```python
from build123d import *

# Parameters (mm, degrees)
F1_DEPTH = 43


with BuildPart() as f1:
    # F0 (on Top) → F1 (new body)
    with BuildSketch(Plane.XY):
        with BuildLine():
            Line((-14, 11), (-14, -7))
            Line((-14, -7), (-7, -14))
            Line((-7, -14), (0, -14))
            Line((0, -14), (21.066626, -14))
            ThreePointArc((21.066626, -14), (24.331862, -15.213414), (26.012265, -18.264706))
            ThreePointArc((26.012265, -18.264706), (28.349095, -26.115672), (32.788067, -33))
            Line((32.788067, -33), (38, -33))
            Line((38, -33), (67, 0))
            Line((67, 0), (67, 19))
            Line((67, 19), (62, 24))
            Line((62, 24), (38, 24))
            ThreePointArc((38, 24), (29.574973, 16.276069), (18.243085, 14.783252))
            Line((18.243085, 14.783252), (0, 18))
            Line((0, 18), (-7, 18))
            Line((-7, 18), (-14, 11))
        make_face()
        with BuildLine():
            ThreePointArc((7, 0), (4.949747, -4.949747), (0, -7))
            ThreePointArc((0, -7), (-4.949747, 4.949747), (7, 0))
        make_face(mode=Mode.SUBTRACT)
    extrude(amount=F1_DEPTH)


solid = f1.part
```
Build history of the part. All positions in model axes, mm. A direction names the side the tool comes from. Coordinates: 2 decimals unless noted, no trailing zeros. Order: outer loops, then holes, each group sorted by start corner. A loop starts at its lowest first (then second) coordinate and runs counter-clockwise, first axis right, second up. Notation, with made-up numbers: (49.25, 79.5) -> (62.25, 79.5) arc R33 cw to (62.25, 108.5) -> close; hole circle Ø11 at (49, 6.25). An arc over 180 degrees is marked (long way). Answer in a Markdown table with one row per item. Add a question column.
Q1. Band-saw the part on D-D, the plane x = 52.5. List the corners of the cut face in (y, z), then the cut area to 3 significant figures.
Q2. Band-saw the part on A-A, the plane z = 3. List the corners of the cut face in (x, y).
Q3. Drop flat-ended pins along their axis: pin 1 (3 mm diameter, centred on y = -6.5, z = 11.5, fed in from +X); pin 2 (3 mm diameter, centred on y = -26.5, z = 8, fed in from +X); pin 3 (10 mm diameter, centred on x = 12.5, z = 5, fed in from +Y); pin 4 (18 mm diameter, centred on x = 0, y = 0, fed in from +Z). Give the stop position or say it passes through.
Q4. Band-saw the part on C-C, the plane x = 6. List the corners of the cut face in (y, z), then the cut area to 3 significant figures.
Q5. Wall check: line 1 along Y through (x, z) = (0, 12); line 2 along Y through (x, z) = (0.5, 34.5); line 3 along X through (y, z) = (1, 35.5). Give the ranges that are in metal, low to high. Write a range as [from, to].
Q6. Band-saw the part on B-B, the plane y = -6. List the corners of the cut face in (x, z), then the cut area to 3 significant figures.
Q7. Which spindle directions (+Z, -Z, +X, -X, +Y, -Y) get a long thin tool onto all of the face, cutting with end or side? Do faces 1 (the face through (-14, 2, 21)), 2 (the face through (-3, 18, 21)), 3 (the face through (52.3, -16.73, 21.2)), 4 (the face through (9.25, 16.37, 21.2)), 5 (the face through (7, -14, 21)). Say none if no direction does.
Q8. Mould opens along X. For faces 6 (the face through (26, 2, 43)), 7 (the face through (24.29, -15.18, 21.2)), 8 (the face through (29.722, 16.345, 21.199)) say: +X half, -X half, draft (parallel to the pull), parting line (faces both ways), or undercut.
Answers follow:
| question | item | result |
|---|---|---|
| 1 | outline | (-16.5, 0) -> (24, 0) -> (24, 43) -> (-16.5, 43) -> close |
| 1 | area | 1,740 mm^2 |
| 2 | outline | (-14, -7) -> (-7, -14) -> (21.07, -14) arc R5 cw to (26.01, -18.26) arc R29 ccw to (32.79, -33) -> (38, -33) -> (67, 0) -> (67, 19) -> (62, 24) -> (38, 24) arc R19 cw to (18.24, 14.78) -> (0, 18) -> (-7, 18) -> (-14, 11) -> close; hole (0, -7) arc R7 ccw to (7, 0) arc R7 ccw (long way) to start |
| 3 | pin 1 | x = 62.61 |
| 3 | pin 2 | x = 45.03 |
| 3 | pin 3 | y = 16.68 |
| 3 | pin 4 | z = 43 |
| 4 | outline | (-14, 0) -> (-3.61, 0) -> (-3.61, 43) -> (-14, 43) -> close; (3.61, 0) -> (16.94, 0) -> (16.94, 43) -> (3.61, 43) -> close |
| 4 | area | 1,020 mm^2 |
| 5 | line 1 | [-14, -7], [7, 18] |
| 5 | line 2 | [-14, -6.98], [6.98, 17.91] |
| 5 | line 3 | [-14, -6.93], [6.93, 67] |
| 6 | outline | (-14, 0) -> (-3.61, 0) -> (-3.61, 43) -> (-14, 43) -> close; (3.61, 0) -> (61.73, 0) -> (61.73, 43) -> (3.61, 43) -> close |
| 6 | area | 2,950 mm^2 |
| 7 | face 1 | +Z, -Z, -X, +Y, -Y |
| 7 | face 2 | +Z, -Z, -X, +Y |
| 7 | face 3 | +Z, -Z, +X, -Y |
| 7 | face 4 | +Z, -Z, +Y |
| 7 | face 5 | +Z, -Z, -X, -Y |
| 8 | face 6 | draft |
| 8 | face 7 | -X half |
| 8 | face 8 | undercut |
